from build123d import *

# Parameters (mm, degrees)
BOX009_W          = 5
BOX009_H          = 24
BOX009_DEPTH      = 40
BOX009_ROLL_ANGLE = -2.2
BOX008_W          = 5
BOX008_H          = 25
BOX008_DEPTH      = 38
FILLET046_R       = 3


with BuildPart() as cube080:
    # Box009 → Box009 (new body)
    with BuildSketch(Plane.XY):
        with Locations((2.5, 12)):
            Rectangle(BOX009_W, BOX009_H)
    extrude(amount=BOX009_DEPTH)


with BuildPart() as cube080_1:
    # Box009 roll: moved
    add(cube080.part.rotate(Axis((0, 0, 0), (1, 0, 0)), BOX009_ROLL_ANGLE))


with BuildPart() as cube080_2:
    # Box009 placement: moved
    add(cube080_1.part.moved(Location((175, -24, -1))))


with BuildPart() as cut003:
    # Box008 → Box008 (new body)
    with BuildSketch(Plane(origin=(175, 0, 0), x_dir=(1, 0, 0), z_dir=(0, 0, 1))):
        with Locations((2.5, 12.5)):
            Rectangle(BOX008_W, BOX008_H)
    extrude(amount=BOX008_DEPTH)

    # Cut003: cut Cube080
    add(cube080_2.part, mode=Mode.SUBTRACT)


with BuildPart() as cut003_1:
    # Cut003 placement: moved
    add(cut003.part.moved(Location((0, 1, 1))))


with BuildPart() as fillet046:
    # Part__Mirroring001: instance of Cut003
    add(cut003_1.part.mirror(Plane(origin=(0, 0, 0), x_dir=(1, 0, 0), z_dir=(0, 1, 0))))


with BuildPart() as fillet046_1:
    # Part__Mirroring001 placement: moved
    add(fillet046.part.moved(Location((-57, 154, 73))))

    # Fillet046
    fillet046_edges = [fillet046_1.edges().sort_by_distance(p)[0] for p in [
        (120.5, 128, 74),
        (120.5, 128, 112),
        (120.5, 152.943881, 74),
        (120.5, 151.484068, 112),
    ]]
    fillet(fillet046_edges, radius=FILLET046_R)


solid = fillet046_1.part
Build history of the part. All positions in model axes, mm. Coordinates: 2 decimals unless noted, no trailing zeros. Order: outer loops, then holes, each group sorted by start corner. A loop starts at its lowest first (then second) coordinate and runs counter-clockwise, first axis right, second up. Notation, with made-up numbers: (46.25, 76) - (51.25, 76) arc R15 ccw to (51.25, 88) - close; hole circle Ø11 at (30.5, 18). An arc over 180 degrees is marked (long way). Write each question's results on one line, items separated by ' | '. Start each with the question number.
Item 1: Band-saw the part on B-B on z = 107.5. Write the cut outline in (x, y), and give its area (3 significant figures).
Item 2: Flat gauge pins, fed straight in: pin 1 (1.5 mm diameter, centred on x = 119.5, z = 100, fed in from +Y); pin 2 (1.5 mm diameter, centred on x = 121, z = 89, fed in from +Y). Where does each tip first touch, or does it go through?
Item 3: Band-saw the part on A-A on x = 121. Write the cut outline in (y, z), and give its area (3 significant figures).
Item 4: Band-saw the part on C-C on z = 102.5. Write the cut outline in (x, y).
Item 5: Wall check: probe 1 along Y at (x, z) = (121.85, 92.5); probe 2 along Y at (x, z) = (121.4, 84); probe 3 along Z at (x, y) = (118.2, 148.75). Give the ranges that are in metal, low to high. Write a range as [from, to].
Numbers:
1) outline: (118, 128) - (123, 128) - (123, 151.66) - (118, 151.66) - close | area: 118 mm^2
2) pin 1: y = 151.97 | pin 2: y = 152.4
3) outline: (128, 77) arc R3 ccw to (131, 74) - (149.83, 74) arc R3 ccw to (152.82, 77.12) - (151.59, 109.12) arc R3 ccw to (148.6, 112) - (131, 112) arc R3 ccw to (128, 109) - close | area: 912 mm^2
4) outline: (118, 128) - (123, 128) - (123, 151.85) - (118, 151.85) - close
5) probe 1: [128, 152.23] | probe 2: [128, 152.56] | probe 3: [74, 112]
